The listing builds one solid part. Answer for the finished solid, in the listing's coordinates (mm). Face numbers are marked on the shaded views. A direction names the side the tool comes from. Give positions to 0.01 mm unless a question says otherwise; leave off trailing zeros. Order: outer loops, then holes, each group sorted by start corner. A loop starts at its lowest first (then second) coordinate and runs counter-clockwise, first axis right, second up. Notation, with made-up numbers: (42.5, 8.25) - (63.5, 8.25) arc R32 cw to (63.5, 41.25) - close; hole circle Ø5 at (31.25, 81). An arc over 180 degrees is marked (long way). Answer in a Markdown table with one row per item.
Autodesk Inventor part; units mm, degrees
ref_plane "YZ Plane" through (0, 0, 0) normal (1, 0, 0) x (0, 1, 0)
ref_plane "XZ Plane" through (0, 0, 0) normal (0, 1, 0) x (-1, 0, 0)
ref_plane "XY Plane" through (0, 0, 0) normal (0, 0, 1) x (1, 0, 0)
sketch "Sketch1" plane through (0, 0, 0) normal (0, 0, 1) x (1, 0, 0)
  arc A0 (241.112, 10.0687) -> (56.7808, 234.547) centre (0, 0) ccw
  arc A1 (215.712, 9.008) -> (50.7992, 209.8386) centre (0, 0) ccw
  line L0 (241.112, 10.0687) -> (215.712, 9.008)
  line L1 (56.7808, 234.547) -> (50.7992, 209.8386)
  line L2 (56.7808, 234.547) -> (0, 0) construction
  line L3 (0, 0) -> (241.112, 10.0687) construction
  point P0 (0, 0)
  dimension "d0" = 74
  dimension "d1" = 25.4
  dimension "d2" = 215.9
extrude "Extrusion1" add sketch "Sketch1" along normal blind 25.4
shell "Shell1" thickness 1.5875 removed faces 2 at (232.6453, 9.7152, 8.4667) at (52.7931, 218.0748, 8.4667)
sketch "Sketch2" plane through (0, 0, 25.4) normal (0, 0, 1) x (1, 0, 0)
  line L0 (50.7992, 209.8386) -> (56.7808, 234.547)
  arc A0 (215.712, 9.008) -> (50.7992, 209.8386) centre (0, 0) ccw
  line L1 (56.7808, 234.547) -> (50.7992, 209.8386)
  arc A1 (76.1992, 202.0062) -> (50.7992, 209.8386) centre (0, 0) ccw
  arc A2 (85.1716, 225.7923) -> (56.7808, 234.547) centre (0, 0) ccw
  line L2 (76.1992, 202.0062) -> (85.1716, 225.7923)
  line L3 (0, 0) -> (76.1992, 202.0062) construction
  line L4 (50.7992, 209.8386) -> (76.1992, 202.0062) construction
  dimension "d6" = 25.4
extrude "Extrusion2" cut sketch "Sketch2" against normal through all
properties part number "Frame_BottomGuideRail"
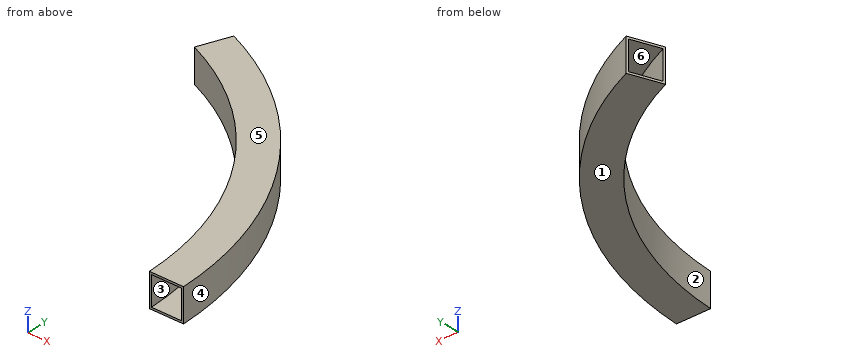
Item 1: Find section D-D on x = 224.5. Write down the section's boundary in (y, z), then the cut area to 3 significant figures.
Answer block:
| item | result |
|---|---|
| outline | (9.37, 0) - (88.52, 0) - (88.52, 25.4) - (9.37, 25.4) - (9.37, 23.81) - (84.1, 23.81) - (84.1, 1.59) - (9.37, 1.59) - close |
| area | 350 mm² |
Item 2: Consider line 1 (Z direction, x = 203, y = 80); line 2 (X direction, y = 135, z = 10.25); line 3 (X direction, y = 138, z = 22.75). Determine where each line is inside the solid, lowest interval first.
Answer block:
| item | result |
|---|---|
| line 1 | 0 to 1.59, 23.81 to 25.4 |
| line 2 | 168.49 to 170.52, 198.11 to 200.03 |
| line 3 | 166.04 to 168.1, 196.03 to 197.97 |
Item 3: Find section C-C on z = 8.5. Write down the section's boundary in (x, y).
Answer block:
| item | result |
|---|---|
| outline | (76.2, 202.01) arc R215.9 cw to (215.71, 9.01) - (217.3, 9.07) arc R217.49 ccw to (76.76, 203.49) - close; (84.61, 224.31) arc R239.73 cw to (239.53, 10) - (241.11, 10.07) arc R241.32 ccw to (85.17, 225.79) - close |
Item 4: Determine the mould class of the marked faces 1, 2, 3 and 4 for opening direction X: pulls with the +X half, pulls with the -X half, needs draft (parallel to the pull), parting line crosses it, or undercut.
Answer block:
| item | result |
|---|---|
| face 1 | needs draft |
| face 2 | pulls with the -X half |
| face 3 | undercut |
| face 4 | pulls with the +X half |
Item 5: Each of these flat-tipped pins is pushed along its axis until it touches: P1, Ø6, axis at x = 172.5, z = 17, coming from the +Y side; P2, Ø6, axis at y = 57, z = 5, coming from the -X side; P3, Ø5, axis at y = 46.5, z = 21.5, coming from the +X side. Where does it stop, or does it pass through?
Answer block:
| item | result |
|---|---|
| P1 | y = 171.77 |
| P2 | x = 207.4 |
| P3 | x = 237.28 |
Item 6: Which of the six approach directions +Z, -Z, +X, -X, +Y, -Y give full straight-line access (tool end or side, diameter ignored) to the marked faces 5 and 6?
Answer block:
| item | result |
|---|---|
| face 5 | +Z, +X, -X, +Y, -Y |
| face 6 | none |
Item 7: Find section A-A on y = 190. Write down the section's boundary in (x, z).
Answer block:
| item | result |
|---|---|
| outline | (102.53, 0) - (148.78, 0) - (148.78, 25.4) - (102.53, 25.4) - close; hole (105.83, 1.59) - (146.19, 1.59) - (146.19, 23.81) - (105.83, 23.81) - close |
Item 8: Find section B-B on x = 206. Write down the section's boundary in (y, z).
Answer block:
| item | result |
|---|---|
| outline | (64.63, 0) - (125.7, 0) - (125.7, 25.4) - (64.63, 25.4) - close; hole (69.75, 1.59) - (122.62, 1.59) - (122.62, 23.81) - (69.75, 23.81) - close |
